```python
from build123d import *

# Parameters (mm, degrees)
SKETCH_1_W          = 96
SKETCH_1_H          = 62
EXTRUDE_1_DEPTH     = 5
SKETCH_2_W          = 96
SKETCH_2_H          = 62
SKETCH_2_W_2        = 91.6
SKETCH_2_H_2        = 57.6
CUT_EXTRUDE_1_DEPTH = 2
EXTRUDE_2_DEPTH     = 3
FILLET_1_R          = 3
FILLET_2_R          = 1
FILLET_3_R          = 0.6
FILLET_4_R          = 0.6
SKETCH_5_R          = 2.25
CUT_EXTRUDE_2_DEPTH = 2
SKETCH_6_R          = 2.25
SKETCH_6_W          = 5
SKETCH_6_H          = 5
SKETCH_6_R_2        = 2.75
SKETCH_6_W_2        = 8
SKETCH_6_H_2        = 6
CUT_EXTRUDE_3_DEPTH = 63.465990747


with BuildPart() as part:
    # Эскиз1 → Бобышка-Вытянуть1 (new body)
    with BuildSketch(Plane(origin=(0, 0, 0), x_dir=(1, 0, 0), z_dir=(0, 1, 0))):
        Rectangle(SKETCH_1_W, SKETCH_1_H)
    extrude(amount=EXTRUDE_1_DEPTH)

    # Эскиз2 → Вырез-Вытянуть1 (cut)
    with BuildSketch(Plane(origin=(0, 5, 0), x_dir=(1, 0, 0), z_dir=(0, 1, 0))):
        Rectangle(SKETCH_2_W, SKETCH_2_H)
        Rectangle(SKETCH_2_W_2, SKETCH_2_H_2, mode=Mode.SUBTRACT)
    extrude(amount=-CUT_EXTRUDE_1_DEPTH, mode=Mode.SUBTRACT)

    # Эскиз4 → Бобышка-Вытянуть2 (add)
    with BuildSketch(Plane.XZ):
        with BuildLine():
            Line((-54, 31), (-54, 24))
            Line((-54, 24), (-51, 24))
            Line((-51, 24), (-51, 26.25))
            ThreePointArc((-51, 26.25), (-51.883883476, 28.383883476), (-49.75, 27.5))
            Line((-49.75, 27.5), (-48, 27.5))
            Line((-48, 27.5), (-48, 31))
            Line((-48, 31), (-54, 31))
        make_face()
        with BuildLine():
            Line((-51, 26.25), (-51, 24))
            Line((-51, 24), (-48, 24))
            Line((-48, 24), (-48, 27.5))
            Line((-48, 27.5), (-49.75, 27.5))
            ThreePointArc((-49.75, 27.5), (-50.116116524, 26.616116524), (-51, 26.25))
        make_face()
        with BuildLine():
            Line((-54, -24), (-54, -31))
            Line((-54, -31), (-48, -31))
            Line((-48, -31), (-48, -27.5))
            Line((-48, -27.5), (-49.75, -27.5))
            ThreePointArc((-49.75, -27.5), (-51.883883476, -28.383883476), (-51, -26.25))
            Line((-51, -26.25), (-51, -24))
            Line((-51, -24), (-54, -24))
        make_face()
        with BuildLine():
            Line((-49.75, -27.5), (-48, -27.5))
            Line((-48, -27.5), (-48, -24))
            Line((-48, -24), (-51, -24))
            Line((-51, -24), (-51, -26.25))
            ThreePointArc((-51, -26.25), (-50.116116524, -26.616116524), (-49.75, -27.5))
        make_face()
        with BuildLine():
            Line((48, -27.5), (48, -31))
            Line((48, -31), (54, -31))
            Line((54, -31), (54, -24))
            Line((54, -24), (51, -24))
            Line((51, -24), (51, -26.25))
            ThreePointArc((51, -26.25), (51.883883476, -26.616116524), (52.25, -27.5))
            ThreePointArc((52.25, -27.5), (51, -28.75), (49.75, -27.5))
            Line((49.75, -27.5), (48, -27.5))
        make_face()
        with BuildLine():
            Line((48, -24), (48, -27.5))
            Line((48, -27.5), (49.75, -27.5))
            ThreePointArc((49.75, -27.5), (50.116116524, -26.616116524), (51, -26.25))
            Line((51, -26.25), (51, -24))
            Line((51, -24), (48, -24))
        make_face()
        with BuildLine():
            Line((51, 24), (54, 24))
            Line((54, 24), (54, 31))
            Line((54, 31), (48, 31))
            Line((48, 31), (48, 27.5))
            Line((48, 27.5), (49.75, 27.5))
            ThreePointArc((49.75, 27.5), (51, 28.75), (52.25, 27.5))
            ThreePointArc((52.25, 27.5), (51.883883476, 26.616116524), (51, 26.25))
            Line((51, 26.25), (51, 24))
        make_face()
        with BuildLine():
            Line((48, 27.5), (48, 24))
            Line((48, 24), (51, 24))
            Line((51, 24), (51, 26.25))
            ThreePointArc((51, 26.25), (50.116116524, 26.616116524), (49.75, 27.5))
            Line((49.75, 27.5), (48, 27.5))
        make_face()
    extrude(amount=-EXTRUDE_2_DEPTH)

    # Скругление1
    fillet_1_edges = [part.edges().sort_by_distance(p)[0] for p in [
        (-48, 1.5, 24),
        (-48, 1.5, -24),
        (48, 1.5, -24),
        (48, 1.5, 24),
    ]]
    fillet(fillet_1_edges, radius=FILLET_1_R)

    # Скругление2
    fillet_2_edges = [part.edges().sort_by_distance(p)[0] for p in [
        (-54, 1.5, 24),
        (-54, 1.5, 31),
        (-54, 1.5, -31),
        (-54, 1.5, -24),
        (54, 1.5, -24),
        (54, 1.5, -31),
        (54, 1.5, 31),
        (54, 1.5, 24),
    ]]
    fillet(fillet_2_edges, radius=FILLET_2_R)

    # Скругление3
    fillet_3_edges = [part.edges().sort_by_distance(p)[0] for p in [
        (45.8, 5, 0),
        (0, 5, 28.8),
        (-45.8, 5, 0),
        (0, 5, -28.8),
    ]]
    fillet(fillet_3_edges, radius=FILLET_3_R)

    # Скругление4
    # the kernel refuses this fillet: 0.6 mm, written as the material it takes off along each edge
    with BuildSketch(Plane(origin=(-45.2, 4.4, -28.2), x_dir=(0, 0, -1), z_dir=(-1, 0, 0))) as fillet_4_piece_1_section:
        Polygon((0, 0), (FILLET_4_R * 1.02, 0), (FILLET_4_R * 1.02, -FILLET_4_R * 1.02), (0, -FILLET_4_R * 1.02), align=None)
    fillet_4_piece_1 = extrude(amount=FILLET_4_R * 1.02, mode=Mode.PRIVATE)
    fillet_4_piece_1 = fillet_4_piece_1 - Plane(origin=(-45.2, 4.4, -28.2), x_dir=(0, -0.7071067811865475, 0.7071067811865475), z_dir=(-1, 0, 0)) * Sphere(FILLET_4_R, mode=Mode.PRIVATE)
    add(fillet_4_piece_1, mode=Mode.SUBTRACT)
    with BuildSketch(Plane(origin=(45.2, 4.4, -28.2), x_dir=(1, 0, 0), z_dir=(0, 0, -1))) as fillet_4_piece_2_section:
        Polygon((0, 0), (FILLET_4_R * 1.02, 0), (FILLET_4_R * 1.02, -FILLET_4_R * 1.02), (0, -FILLET_4_R * 1.02), align=None)
    fillet_4_piece_2 = extrude(amount=FILLET_4_R * 1.02, mode=Mode.PRIVATE)
    fillet_4_piece_2 = fillet_4_piece_2 - Plane(origin=(45.2, 4.4, -28.2), x_dir=(-0.7071067811865475, -0.7071067811865475, 0), z_dir=(0, 0, -1)) * Sphere(FILLET_4_R, mode=Mode.PRIVATE)
    add(fillet_4_piece_2, mode=Mode.SUBTRACT)
    with BuildSketch(Plane(origin=(-45.2, 4.4, 28.2), x_dir=(0, 0, 1), z_dir=(-1, 0, 0))) as fillet_4_piece_3_section:
        Polygon((0, 0), (FILLET_4_R * 1.02, 0), (FILLET_4_R * 1.02, FILLET_4_R * 1.02), (0, FILLET_4_R * 1.02), align=None)
    fillet_4_piece_3 = extrude(amount=FILLET_4_R * 1.02, mode=Mode.PRIVATE)
    fillet_4_piece_3 = fillet_4_piece_3 - Plane(origin=(-45.2, 4.4, 28.2), x_dir=(0, -0.7071067811865475, -0.7071067811865475), z_dir=(-1, 0, 0)) * Sphere(FILLET_4_R, mode=Mode.PRIVATE)
    add(fillet_4_piece_3, mode=Mode.SUBTRACT)
    with BuildSketch(Plane(origin=(45.2, 4.4, 28.2), x_dir=(1, 0, 0), z_dir=(0, 0, 1))) as fillet_4_piece_4_section:
        Polygon((0, 0), (FILLET_4_R * 1.02, 0), (FILLET_4_R * 1.02, FILLET_4_R * 1.02), (0, FILLET_4_R * 1.02), align=None)
    fillet_4_piece_4 = extrude(amount=FILLET_4_R * 1.02, mode=Mode.PRIVATE)
    fillet_4_piece_4 = fillet_4_piece_4 - Plane(origin=(45.2, 4.4, 28.2), x_dir=(-0.7071067811865475, -0.7071067811865475, 0), z_dir=(0, 0, 1)) * Sphere(FILLET_4_R, mode=Mode.PRIVATE)
    add(fillet_4_piece_4, mode=Mode.SUBTRACT)
    with BuildSketch(Plane(origin=(45.8, 4.4, 28.8), x_dir=(-1, 0, 0), z_dir=(0, -1, 0)), Plane(origin=(-45.8, 4.4, 28.8), x_dir=(0, 0, -1), z_dir=(0, -1, 0))) as fillet_4_piece_5:
        with BuildLine():
            CenterArc((FILLET_4_R, FILLET_4_R), FILLET_4_R, 180, 90)
            Line((0, FILLET_4_R), (0, 0))
            Line((0, 0), (FILLET_4_R, 0))
        make_face()
    extrude(amount=1.4, mode=Mode.SUBTRACT)
    with BuildSketch(Plane(origin=(-45.8, 4.4, -28.8), x_dir=(0, 0, 1), z_dir=(0, -1, 0)), Plane(origin=(45.8, 4.4, -28.8), x_dir=(-1, 0, 0), z_dir=(0, -1, 0))) as fillet_4_piece_6:
        with BuildLine():
            CenterArc((FILLET_4_R, -FILLET_4_R), FILLET_4_R, 90, 90)
            Line((0, -FILLET_4_R), (0, 0))
            Line((0, 0), (FILLET_4_R, 0))
        make_face()
    extrude(amount=1.4, mode=Mode.SUBTRACT)

    # Эскиз5 → Вырез-Вытянуть2 (cut)
    with BuildSketch(Plane.XZ):
        with Locations(Location((-51, 27.5, 0), (0, 0, 270))):
            Circle(SKETCH_5_R)
        with Locations(Location((51, 27.5, 0), (0, 0, 270))):
            Circle(SKETCH_5_R)
        with Locations(Location((-51, -27.5, 0), (0, 0, 270))):
            Circle(SKETCH_5_R)
        with Locations(Location((51, -27.5, 0), (0, 0, 270))):
            Circle(SKETCH_5_R)
    extrude(amount=-CUT_EXTRUDE_2_DEPTH, mode=Mode.SUBTRACT)

    # Эскиз6 → Вырез-Вытянуть3 (cut, through all)
    with BuildSketch(Plane.XZ):
        with Locations(Location((-28.5, 4.5, 0), (0, 0, 270))):
            Circle(SKETCH_6_R)
        with Locations((-21, 4.5)):
            Rectangle(SKETCH_6_W, SKETCH_6_H)
        with Locations(Location((25.33, -4, 0), (0, 0, 270))):
            Circle(SKETCH_6_R_2)
        with Locations(Location((32.93, -4, 0), (0, 0, 270))):
            Circle(SKETCH_6_R_2)
        with Locations(Location((32.93, 3.75, 0), (0, 0, 270))):
            Circle(SKETCH_6_R_2)
        with Locations(Location((25.33, 3.75, 0), (0, 0, 270))):
            Circle(SKETCH_6_R_2)
        with Locations((25.3, -11.5)):
            Rectangle(SKETCH_6_W_2, SKETCH_6_H_2)
        with Locations((25.3, -22.4)):
            Rectangle(SKETCH_6_W_2, SKETCH_6_H_2)
        with Locations((38, -22.4)):
            Rectangle(SKETCH_6_W_2, SKETCH_6_H_2)
        with Locations((38, -11.5)):
            Rectangle(SKETCH_6_W_2, SKETCH_6_H_2)
    extrude(amount=-CUT_EXTRUDE_3_DEPTH, mode=Mode.SUBTRACT)


solid = part.part
```
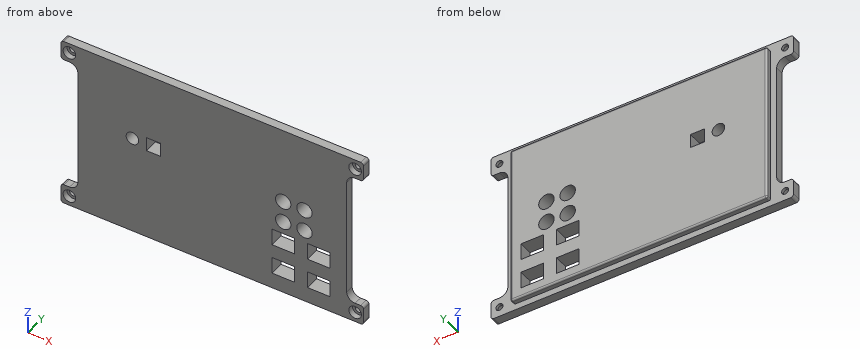
Model file for the job. Use its own axes, mm. Round coordinates to 2 decimals unless told otherwise and drop trailing zeros. Write each loop counter-clockwise with the first axis right and the second up, starting at its lowest first coordinate (ties: lowest second). Pieces come first, ordered by that corner, then holes. Notation, with made-up numbers: M -6.5,-30.5 L 15.5,-30.5 A16 ccw 15.5,-26.5 Z; hole C 60,89 d7. An arc over 180 degrees is marked long. Put each result on its own line as item: value.
Item 1: Cut at D-D (x = 12). List the corners of the cut face in (y, z).
Responses:
outline: M 0,-31 L 3,-31 L 3,-28.8 L 4.4,-28.8 A0.6 ccw 5,-28.2 L 5,28.2 A0.6 ccw 4.4,28.8 L 3,28.8 L 3,31 L 0,31 Z
Item 2: Cut at A-A (x = 32.93). List the corners of the cut face in (y, z), and give its area (3 significant figures).
Responses:
outline: M 0,-31 L 3,-31 L 3,-28.8 L 4.4,-28.8 A0.6 ccw 5,-28.2 L 5,-6.75 L 0,-6.75 Z; M 0,-1.25 L 5,-1.25 L 5,1 L 0,1 Z; M 0,6.5 L 5,6.5 L 5,28.2 A0.6 ccw 4.4,28.8 L 3,28.8 L 3,31 L 0,31 Z
area: 246 mm²
Item 3: Cut at C-C (z = 3.75). List the corners of the cut face in (x, y).
Responses:
outline: M -48,0 L -30.62,0 L -30.62,5 L -45.2,5 A0.6 ccw -45.8,4.4 L -45.8,3 L -48,3 Z; M -26.38,0 L -23.5,0 L -23.5,5 L -26.38,5 Z; M -18.5,0 L 22.58,0 L 22.58,5 L -18.5,5 Z; M 28.08,0 L 30.18,0 L 30.18,5 L 28.08,5 Z; M 35.68,0 L 48,0 L 48,3 L 45.8,3 L 45.8,4.4 A0.6 ccw 45.2,5 L 35.68,5 Z
Item 4: Flat gauge pins, fed straight in: P1, Ø1.5, axis at y = 1.5, z = -12.5, coming from the -X side; P2, Ø6, axis at x = 51, z = -27.5, coming from the +Y side; P3, Ø1.5, axis at x = -51, z = -27.5, coming from the +Y side. Where does each tip first touch, or does it go through?
Responses:
P1: x = -48
P2: y = 3
P3: through
Item 5: Probe L1, parallel to Z at x = -51, y = 2.5; L2, parallel to X at y = 1.55, z = 27.5; L3, parallel to Z at x = 37, y = 4.5. List the from-to ranges inside material, lowest first. Write a range as from..to.
Responses:
L1: -31..-28.75, -26.25..-24, 24..26.25, 28.75..31
L2: -54..-53.25, -48.75..48.75, 53.25..54
L3: -28.79..-25.4, -19.4..-14.5, -8.5..28.79
Item 6: Cut at B-B (z = -11). List the corners of the cut face in (x, y), and give its area (3 significant figures).
Responses:
outline: M -48,0 L 21.3,0 L 21.3,5 L -45.2,5 A0.6 ccw -45.8,4.4 L -45.8,3 L -48,3 Z; M 29.3,0 L 34,0 L 34,5 L 29.3,5 Z; M 42,0 L 48,0 L 48,3 L 45.8,3 L 45.8,4.4 A0.6 ccw 45.2,5 L 42,5 Z
area: 391 mm²
